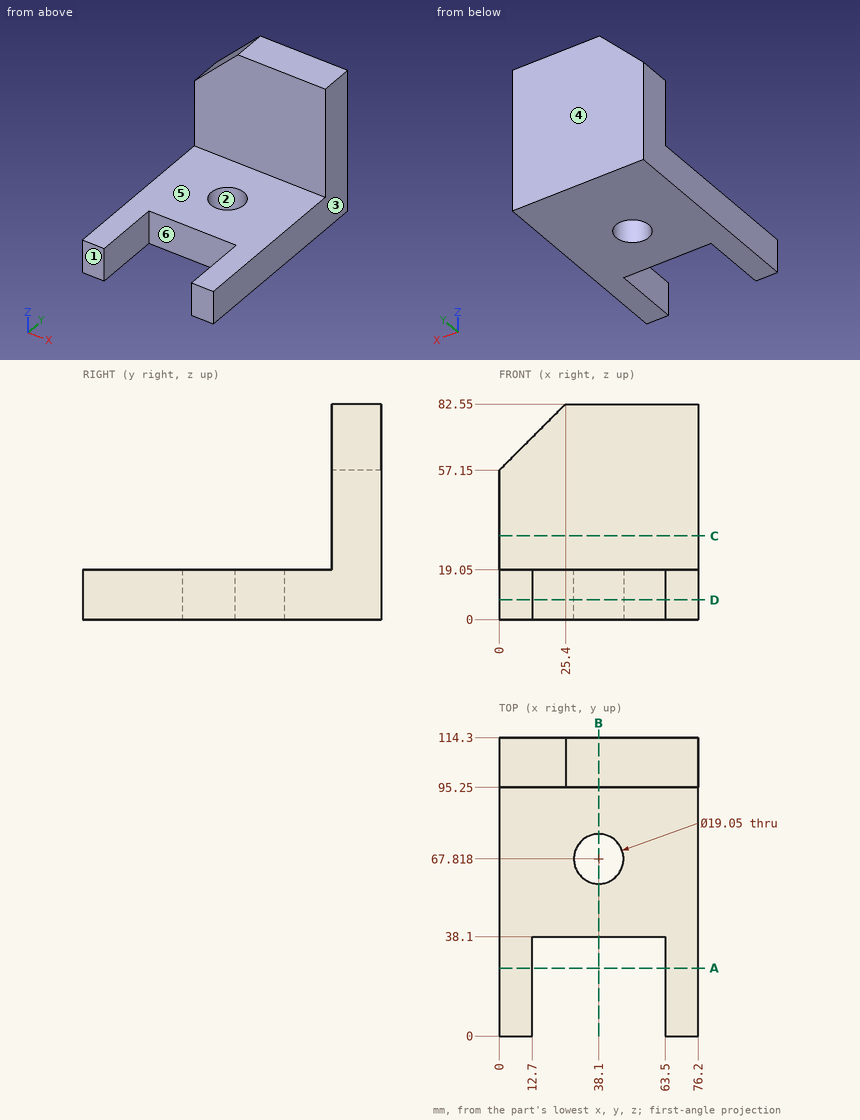
Geometry check sheet. Reference: drawing and pictorial views, mm from the part's lowest x, y, z. A direction names the side the tool comes from. Round coordinates to 2 decimals unless told otherwise and drop trailing zeros. Loops run counter-clockwise (first coordinate to the right, second up) from the corner with the lowest first, then second, coordinate; pieces in that order, holes last. Notation, with made-up numbers: (73, 4.5) - (78, 4.5) arc R6 cw to (78, 10.5) - close; hole circle Ø10 at (2.5, -17). An arc over 180 degrees is marked (long way). Use a Markdown table: item, result. Add a question column.
1. Access from +Z, -Z, +X, -X, +Y, -Y to the whole of each face (thin tool, end or side, straight path). Record for the marked faces 4, 5 and 6.
2. Thickness scan on probe 1 along Y at (x, z) = (38.1, 10.5); probe 2 along Z at (x, y) = (67, 65); probe 3 along Y at (x, z) = (11, 35). Record the ranges inside material, lowest first. Write a range as [from, to].
3. Section check D-D, the plane z = 7.5. Record the boundary of the cut face in (x, y) (3 decimals), plus the area to 3 significant figures.
4. Gauge pin test, flat ends, axial feed: pin 1 (5 mm diameter, centred on x = 26, y = 37, fed in from +Z); pin 2 (5.5 mm diameter, centred on x = 36.5, z = 13, fed in from -Y); pin 3 (3 mm diameter, centred on x = 43.5, z = 39.5, fed in from -Y); pin 4 (21 mm diameter, centred on y = 22, z = 12, fed in from -X). Record the tip position at first contact, or that the pin passes through.
5. Section check C-C, the plane z = 32. Record the boundary of the cut face in (x, y), plus the area to 3 significant figures.
6. Release check for a two-part mould opening along X. For the marked faces 1, 2 and 3 record: released by +X, released by -X, zero draft, split by the parting line, or undercut.
7. Section check B-B, the plane x = 38.1. Record the boundary of the cut face in (y, z).
8. Section check A-A, the plane y = 26. Record the boundary of the cut face in (x, z).
Checks:
| question | item | result |
|---|---|---|
| 1 | face 4 | +Z, -Z, +X, -X, +Y |
| 1 | face 5 | +Z, +X, -X, -Y |
| 1 | face 6 | +Z, -Z, -Y |
| 2 | probe 1 | y = [38.1, 58.29], [77.34, 114.3] |
| 2 | probe 2 | z = [0, 19.05] |
| 2 | probe 3 | y = [95.25, 114.3] |
| 3 | outline | (0, 0) - (12.7, 0) - (12.7, 38.1) - (63.5, 38.1) - (63.5, 0) - (76.2, 0) - (76.2, 114.3) - (0, 114.3) - close; hole circle Ø19.05 at (38.1, 67.818) |
| 3 | area | 6,490 mm^2 |
| 4 | pin 1 | stops at z = 19.05 |
| 4 | pin 2 | stops at y = 38.1 |
| 4 | pin 3 | stops at y = 95.25 |
| 4 | pin 4 | stops at x = 0 |
| 5 | outline | (0, 95.25) - (76.2, 95.25) - (76.2, 114.3) - (0, 114.3) - close |
| 5 | area | 1,450 mm^2 |
| 6 | face 1 | zero draft |
| 6 | face 2 | undercut |
| 6 | face 3 | released by +X |
| 7 | outline | (38.1, 0) - (58.29, 0) - (58.29, 19.05) - (38.1, 19.05) - close; (77.34, 0) - (114.3, 0) - (114.3, 82.55) - (95.25, 82.55) - (95.25, 19.05) - (77.34, 19.05) - close |
| 8 | outline | (0, 0) - (12.7, 0) - (12.7, 19.05) - (0, 19.05) - close; (63.5, 0) - (76.2, 0) - (76.2, 19.05) - (63.5, 19.05) - close |
